Autodesk Fusion 360 part; units mm, degrees
sketch "Boceto6" plane through (0, 0, 0) normal (0, 0, 1) x (1, 0, 0)
  line L0 (0, 0) -> (60, 0)
  line L1 (60, 0) -> (60, -100)
  line L2 (0, 0) -> (0, -100)
  line L3 (0, -100) -> (60, -100)
  line L4 (0, 0) -> (60, 0)
  line L5 (60, 0) -> (60, -2)
  line L6 (60, -2) -> (0, -2)
  line L7 (0, -100) -> (0, -98.9254)
  line L8 (0, -100) -> (0, -98)
  line L9 (0, -98) -> (60, -98)
  line L10 (30, 0) -> (30, -104.8793) construction
  line L11 (50, -51.4397) -> (10, -51.4397) construction
  line L12 (10, -53.4397) -> (50, -53.4397) construction
  line L13 (10, -51.4397) -> (50, -51.4397)
  line L14 (50, -53.4397) -> (10, -53.4397)
  arc A0 (10, -51.4397) -> (10, -53.4397) centre (10, -52.4397) ccw
  arc A1 (50, -53.4397) -> (50, -51.4397) centre (50, -52.4397) ccw
  line L15 (10, -83.4397) -> (50, -83.4397) construction
  arc A2 (10, -81.4397) -> (10, -83.4397) centre (10, -82.4397) ccw
  arc A3 (50, -83.4397) -> (50, -81.4397) centre (50, -82.4397) ccw
  line L16 (50, -81.4397) -> (10, -81.4397) construction
  line L17 (10, -81.4397) -> (50, -81.4397)
  line L18 (50, -83.4397) -> (10, -83.4397)
  line L19 (10, -73.4397) -> (50, -73.4397) construction
  arc A4 (10, -71.4397) -> (10, -73.4397) centre (10, -72.4397) ccw
  arc A5 (50, -73.4397) -> (50, -71.4397) centre (50, -72.4397) ccw
  line L20 (50, -71.4397) -> (10, -71.4397) construction
  line L21 (10, -71.4397) -> (50, -71.4397)
  line L22 (50, -73.4397) -> (10, -73.4397)
  line L23 (10, -63.4397) -> (50, -63.4397) construction
  arc A6 (10, -61.4397) -> (10, -63.4397) centre (10, -62.4397) ccw
  arc A7 (50, -63.4397) -> (50, -61.4397) centre (50, -62.4397) ccw
  line L24 (50, -61.4397) -> (10, -61.4397) construction
  line L25 (10, -61.4397) -> (50, -61.4397)
  line L26 (50, -63.4397) -> (10, -63.4397)
  line L27 (10, -43.4397) -> (50, -43.4397) construction
  arc A8 (10, -41.4397) -> (10, -43.4397) centre (10, -42.4397) ccw
  arc A9 (50, -43.4397) -> (50, -41.4397) centre (50, -42.4397) ccw
  line L28 (50, -41.4397) -> (10, -41.4397) construction
  line L29 (10, -41.4397) -> (50, -41.4397)
  line L30 (50, -43.4397) -> (10, -43.4397)
  line L31 (10, -33.4397) -> (50, -33.4397) construction
  arc A10 (10, -31.4397) -> (10, -33.4397) centre (10, -32.4397) ccw
  arc A11 (50, -33.4397) -> (50, -31.4397) centre (50, -32.4397) ccw
  line L32 (50, -31.4397) -> (10, -31.4397) construction
  line L33 (10, -31.4397) -> (50, -31.4397)
  line L34 (50, -33.4397) -> (10, -33.4397)
  line L35 (10, -23.4397) -> (50, -23.4397) construction
  arc A12 (10, -21.4397) -> (10, -23.4397) centre (10, -22.4397) ccw
  arc A13 (50, -23.4397) -> (50, -21.4397) centre (50, -22.4397) ccw
  line L36 (50, -21.4397) -> (10, -21.4397) construction
  line L37 (10, -21.4397) -> (50, -21.4397)
  line L38 (50, -23.4397) -> (10, -23.4397)
  line L39 (10, -13.4397) -> (50, -13.4397) construction
  arc A14 (10, -11.4397) -> (10, -13.4397) centre (10, -12.4397) ccw
  arc A15 (50, -13.4397) -> (50, -11.4397) centre (50, -12.4397) ccw
  line L40 (50, -11.4397) -> (10, -11.4397) construction
  line L41 (10, -11.4397) -> (50, -11.4397)
  line L42 (50, -13.4397) -> (10, -13.4397)
  dimension "d3" = 60
  dimension "d4" = 100
  dimension "d7" = 2
  dimension "d8" = 2
  dimension "d48" = 1
  dimension "d49" = 40
  dimension "d50" = 2
  dimension "d51" = 40
  dimension "d52" = 2
  dimension "d53" = 2
  dimension "d56" = 0
  dimension "d57" = 40
extrude "Extruir1" add sketch "Boceto6" against normal blind 2 contours L0 L1 L2 L4 L5 L6 | L1 L2 L6 L9 | L1 L2 L3 L7 L8 L9 | L13 L14 A0 A1 | A2 A3 L17 L18 | A4 A5 L21 L22 | A6 A7 L25 L26 | A8 A9 L29 L30 | A10 A11 L33 L34 | A12 A13 L37 L38 | A14 A15 L41 L42
extrude "Extruir2" add sketch "Boceto6" against normal blind 45 contours L0 L1 L2 L4 L5 L6
extrude "Extruir3" add sketch "Boceto6" against normal blind 45 contours L1 L2 L3 L7 L8 L9
fillet "Empalme1" radius 5 1 edges at (60, -99, -45)
fillet "Empalme2" radius 5 2 edges at (60, -1, -45) (0, -99, -45)
fillet "Empalme3" radius 5 1 edges at (0, -1, -45)
sketch "Boceto7" plane through (0, 0, -45) normal (0, 0, -1) x (1, 0, 0)
  line L0 (5, 2) -> (5, 0)
  line L1 (5, 0) -> (55, 0)
  line L2 (55, 0) -> (55, 2)
  line L3 (55, 2) -> (5, 2)
  line L4 (0, 0) -> (0, -2)
  line L5 (0, -2) -> (60, -2)
  line L6 (60, -2) -> (60, 102)
  dimension "d31" = 2
  dimension "d32" = 60
  dimension "d33" = 104
sketch "Boceto8" plane through (0, -42, 0) normal (0, -1, 0) x (1, 0, 0)
  arc A0 (10, -39.5) -> (15, -44.5) centre (15, -39.5) ccw
  line L0 (15, -44.5) -> (47, -44.5)
  arc A1 (47, -44.5) -> (52, -39.5) centre (47, -39.5) ccw
  line L1 (52, -39.5) -> (52, -7.5)
  arc A2 (52, -7.5) -> (47, -2.5) centre (47, -7.5) ccw
  line L2 (47, -2.5) -> (15, -2.5)
  arc A3 (15, -2.5) -> (10, -7.5) centre (15, -7.5) ccw
  line L3 (10, -7.5) -> (10, -15.5)
  line L4 (10, -15.5) -> (6, -15.5)
  line L5 (6, -15.5) -> (6, -31.5)
  line L6 (6, -31.5) -> (10, -31.5)
  line L7 (10, -31.5) -> (10, -39.5)
  circle A4 centre (46.6, -7.9) radius 3
  circle A5 centre (46.6, -39.1) radius 3
  circle A6 centre (15.4, -7.9) radius 3
  circle A7 centre (15.4, -39.1) radius 3
  circle A8 centre (31, -23.5) radius 4.6
  circle A9 centre (15.4, -7.9) radius 1.6
  circle A10 centre (46.6, -7.9) radius 1.6
  circle A11 centre (46.6, -39.1) radius 1.6
  circle A12 centre (15.4, -39.1) radius 1.6
  dimension "d34" = 3.2
  dimension "d35" = 3.2
  dimension "d36" = 3.2
  dimension "d37" = 3.2
extrude "Extruir4" cut sketch "Boceto8" along normal blind 120 and the other way blind 100 contours A9 | A10 | A11 | A12
sketch "Boceto9" plane through (0, 0.2, 0) normal (0, 1, 0) x (-1, 0, 0)
  circle A0 centre (-31, -23.5) radius 11
  circle A1 centre (-31, -23.5) radius 4.6
  circle A2 centre (-31, -23.5) radius 11
  dimension "d42" = 22
extrude "Extruir5" cut sketch "Boceto9" along normal blind 0 and the other way blind 200 contours A0 A2 | A1
extrude "Extruir6" cut sketch "Boceto6" along normal mid plane 20 contours L13 L14 A0 A1 | A2 A3 L17 L18 | A4 A5 L21 L22 | A6 A7 L25 L26 | A8 A9 L29 L30 | A10 A11 L33 L34 | A12 A13 L37 L38 | A14 A15 L41 L42
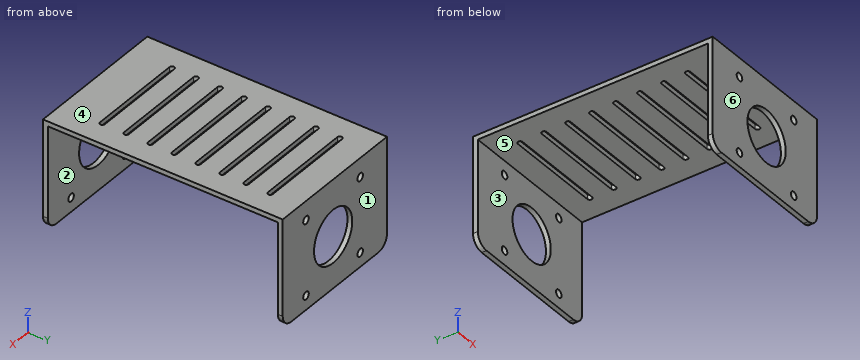
For this review, take the finished solid that the model builds, in its own axes (mm). Face numbers are marked on the shaded views. A direction names the side the tool comes from. Give positions to 0.01 mm unless a question says otherwise; leave off trailing zeros. Write each loop counter-clockwise with the first axis right and the second up, starting at its lowest first coordinate (ties: lowest second). Pieces come first, ordered by that corner, then holes.
Item 1: The part is to be moulded in two halves that separate along Y. For the marked faces 3, 4, 5 and 6, say which applies: +Y half, -Y half, draft (parallel to the pull), parting line (faces both ways), or undercut.
Item 2: Take a section at D-D (x = 31). Give the number of separate pieces and of enclosed holes in the cut face, and give its area (3 significant figures).
Item 3: Take a section at C-C (z = -17.5). Give the boundary of the cut face in (x, y).
Item 4: Machinability: for the marked faces 1 and 2, which of the approach directions +Z, -Z, +X, -X, +Y, -Y give a long, thin tool a straight path to every point of the face, cutting with its end or side? Answer none if there is none.
Item 5: Insertion check: P1, Ø1.6, axis at x = 20, z = -1.5, coming from the +Y side; P2, Ø2.5, axis at x = 15.4, z = -7.9, coming from the +Y side. Each pin has a flat end and moves straight along its axis. Give the tip position at first contact, or say it passes through.
Item 6: Wall thickness on probe 1 along Z at (x, y) = (46.6, -0.5); probe 2 along Z at (x, y) = (31, -1.15); probe 3 along Y at (x, z) = (44.5, -36): over which ranges is each line inside the solid? List them lowest first.
Item 7: Take a section at B-B (x = 52). Give the boundary of the cut face in (y, z).
Item 8: Take a section at A-A (z = -10.5). Give the boundary of the cut face in (x, y), and give its area (3 significant figures).
Established:
1. face 3: undercut
1. face 4: draft
1. face 5: undercut
1. face 6: -Y half
2. separate pieces: 11
2. enclosed holes: 0
2. area: 252 mm2
3. outline: (0, -100) - (21.78, -100) - (21.78, -98) - (0, -98) - close; (0, -2) - (21.78, -2) - (21.78, 0) - (0, 0) - close; (40.22, -100) - (60, -100) - (60, -98) - (40.22, -98) - close; (40.22, -2) - (60, -2) - (60, 0) - (40.22, 0) - close
4. face 1: +Z, -Z, +X, -X, +Y
4. face 2: -Z, +X, -X
5. P1: stops at y = 0
5. P2: passes through
6. probe 1: z = -45 to -40.7, -37.5 to -9.5, -6.3 to 0
6. probe 2: z = -45 to -34.5, -12.5 to 0
6. probe 3: y = -100 to -98, -2 to 0
7. outline: (-100, -45) - (-98, -45) - (-98, -2) - (-2, -2) - (-2, -45) - (0, -45) - (0, 0) - (-100, 0) - close
8. outline: (0, -100) - (60, -100) - (60, -98) - (0, -98) - close; (0, -2) - (60, -2) - (60, 0) - (0, 0) - close
8. area: 240 mm2
